Verification items for the finished model (mm, model axes). A direction names the side the tool comes from. Round coordinates to 2 decimals unless told otherwise and drop trailing zeros. Order: outer loops, then holes, each group sorted by start corner. A loop starts at its lowest first (then second) coordinate and runs counter-clockwise, first axis right, second up. Notation, with made-up numbers: M -1,-22.75 L 55,-22.75 A30 ccw 55,5.25 Z; hole C -1.5,-24 d10. An arc over 180 degrees is marked long. Use one line per item in the form item = value. Start each with the question number.
Item 1: Thickness scan on probe 1 along Z at (x, y) = (-33, 75); probe 2 along Y at (x, z) = (-4.85, 0.15); probe 3 along Y at (x, z) = (-4, 0). Record the ranges inside material, lowest first. Write a range as [from, to].
Item 2: Release check for a two-part mould opening along Z. For faces 5 (the flat face through (15, -19, 0)), 6 (the flat face through (33, 29, 14)), 7 (the flat face through (33, 51, 3.5)), 8 (the flat face through (0, 51, -2.5)) record: +Z half, -Z half, draft (parallel to the pull), parting line (faces both ways), or undercut.
Item 3: Cross-section at D-D on y = -17.5. Enter the section's corners in (x, z), then the cut area to 3 significant figures.
Item 4: Tool access check on faces 1 (the flat face through (-32, 66, 26)), 2 (the flat face through (-34, 73, 14)), 3 (the flat face through (11, 0, 0)), 4 (the flat face through (-15, -19, 0)). Record the directions out of +Z, -Z, +X, -X, +Y, -Y that give a thin tool (end or side, any length) a straight path to the whole face; none if there is none.
Item 5: Cross-section at C-C on z = 22. Enter the section's corners in (x, y).
Item 6: Go/stop test with flat-tipped pins: pin 1 Ø4 at (y, z) = (-15, -1) entering from -X; pin 2 Ø2.5 at (x, y) = (4.85, -24) entering from +Z; pin 3 Ø0.9 at (x, z) = (-33, 11) entering from -Y (3 decimals); pin 4 Ø2 at (x, y) = (-20, -5.5) entering from +Z. Record where each tip stops, or that it passes through.
Item 7: Cross-section at A-A on y = 49.5. Enter the section's corners in (x, z), then the cut area to 3 significant figures.
Item 8: Cross-section at B-B on x = -7.5. Enter the section's corners in (y, z), then the cut area to 3 significant figures.
from build123d import *

# Parameters (mm, degrees)
SKETCH1_R           = 1
SKETCH1_W           = 22
SKETCH1_H           = 44
BOSS_EXTRUDE1_DEPTH = 2.5
BOSS_EXTRUDE2_DEPTH = 34
CUT_EXTRUDE1_REACH  = 128.859
SKETCH3_R           = 1
SKETCH3_W           = 22
SKETCH3_H           = 44


with BuildPart() as part:
    # Sketch1 → Boss-Extrude1 (new, symmetric)
    with BuildSketch(Plane.XY):
        Polygon((-15, -29), (15, -29), (15, -9), (35, 21), (35, 101), (-35, 101), (-35, 21), (-15, -9), align=None)
        with Locations((-4.85, -24)):
            Circle(SKETCH1_R, mode=Mode.SUBTRACT)
        with Locations((4.85, -24)):
            Circle(SKETCH1_R, mode=Mode.SUBTRACT)
        with Locations((4.85, 24)):
            Circle(SKETCH1_R, mode=Mode.SUBTRACT)
        with Locations((-4.85, 24)):
            Circle(SKETCH1_R, mode=Mode.SUBTRACT)
        Rectangle(SKETCH1_W, SKETCH1_H, mode=Mode.SUBTRACT)
    extrude(amount=BOSS_EXTRUDE1_DEPTH, both=True)

    # Sketch2 → Boss-Extrude2 (add)
    with BuildSketch(Plane.XY.offset(-2.5)):
        Polygon((-35, 101), (-35, 21), (-32, 16.5), (-32, 98), (32, 98), (32, 16.5), (35, 21), (35, 101), align=None)
    extrude(amount=BOSS_EXTRUDE2_DEPTH)

    # Cut-Extrude1: up to this face of the body (flat: up to its plane)
    cut_extrude1_end = Plane(part.part.faces().sort_by_distance((35, 61, 14.5))[0])
    # Sketch3 → Cut-Extrude1 (cut, up to the picked face)
    with BuildSketch(Plane.ZY.offset(35), mode=Mode.PRIVATE) as cut_extrude1_sk1:
        with Locations(Location((9.65, 27, 0), (0, 0, 270))):
            Circle(SKETCH3_R)
    cut_extrude1_tool1 = split(extrude(cut_extrude1_sk1.sketch, amount=-CUT_EXTRUDE1_REACH, mode=Mode.PRIVATE), bisect_by=cut_extrude1_end, keep=Keep.BOTH, mode=Mode.PRIVATE)
    # Sketch3 → Cut-Extrude1 (cut, up to the picked face)
    with BuildSketch(Plane.ZY.offset(35), mode=Mode.PRIVATE) as cut_extrude1_sk2:
        with Locations(Location((19.35, 27, 0), (0, 0, 270))):
            Circle(SKETCH3_R)
    cut_extrude1_tool2 = split(extrude(cut_extrude1_sk2.sketch, amount=-CUT_EXTRUDE1_REACH, mode=Mode.PRIVATE), bisect_by=cut_extrude1_end, keep=Keep.BOTH, mode=Mode.PRIVATE)
    # Sketch3 → Cut-Extrude1 (cut, up to the picked face)
    with BuildSketch(Plane.ZY.offset(35), mode=Mode.PRIVATE) as cut_extrude1_sk3:
        with Locations(Location((19.35, 75, 0), (0, 0, 270))):
            Circle(SKETCH3_R)
    cut_extrude1_tool3 = split(extrude(cut_extrude1_sk3.sketch, amount=-CUT_EXTRUDE1_REACH, mode=Mode.PRIVATE), bisect_by=cut_extrude1_end, keep=Keep.BOTH, mode=Mode.PRIVATE)
    # Sketch3 → Cut-Extrude1 (cut, up to the picked face)
    with BuildSketch(Plane.ZY.offset(35), mode=Mode.PRIVATE) as cut_extrude1_sk4:
        with Locations(Location((9.65, 75, 0), (0, 0, 270))):
            Circle(SKETCH3_R)
    cut_extrude1_tool4 = split(extrude(cut_extrude1_sk4.sketch, amount=-CUT_EXTRUDE1_REACH, mode=Mode.PRIVATE), bisect_by=cut_extrude1_end, keep=Keep.BOTH, mode=Mode.PRIVATE)
    # Sketch3 → Cut-Extrude1 (cut, up to the picked face)
    with BuildSketch(Plane.ZY.offset(35), mode=Mode.PRIVATE) as cut_extrude1_sk5:
        with Locations((14.5, 51)):
            Rectangle(SKETCH3_W, SKETCH3_H)
    cut_extrude1_tool5 = split(extrude(cut_extrude1_sk5.sketch, amount=-CUT_EXTRUDE1_REACH, mode=Mode.PRIVATE), bisect_by=cut_extrude1_end, keep=Keep.BOTH, mode=Mode.PRIVATE)
    add(cut_extrude1_tool1.solids().sort_by(Axis((-35, 27, 9.65), (1, 0, 0)))[0], mode=Mode.SUBTRACT)
    add(cut_extrude1_tool2.solids().sort_by(Axis((-35, 27, 19.35), (1, 0, 0)))[0], mode=Mode.SUBTRACT)
    add(cut_extrude1_tool3.solids().sort_by(Axis((-35, 75, 19.35), (1, 0, 0)))[0], mode=Mode.SUBTRACT)
    add(cut_extrude1_tool4.solids().sort_by(Axis((-35, 75, 9.65), (1, 0, 0)))[0], mode=Mode.SUBTRACT)
    add(cut_extrude1_tool5.solids().sort_by(Axis((-35, 51, 14.5), (1, 0, 0)))[0], mode=Mode.SUBTRACT)


solid = part.part
Output values:
q1.probe_1 = [-2.5, 8.65], [10.65, 18.35], [20.35, 31.5]
q1.probe_2 = [-29, -25], [-23, -22], [22, 23], [25, 101]
q1.probe_3 = [-29, -24.53], [-23.47, -22], [22, 23.47], [24.53, 101]
q2.face_5 = draft
q2.face_6 = undercut
q2.face_7 = undercut
q2.face_8 = -Z half
q3.outline = M -15,-2.5 L -11,-2.5 L -11,2.5 L -15,2.5 Z; M 11,-2.5 L 15,-2.5 L 15,2.5 L 11,2.5 Z
q3.area = 40.0 mm2
q4.face_1 = +Z, -Y
q4.face_2 = +X, -X
q4.face_3 = +Z, -Z
q4.face_4 = +Z, -Z, -X, -Y
q5.outline = M -35,21 L -32,16.5 L -32,29 L -35,29 Z; M -35,73 L -32,73 L -32,98 L 32,98 L 32,73 L 35,73 L 35,101 L -35,101 Z; M 32,16.5 L 35,21 L 35,29 L 32,29 Z
q6.pin_1 = -15
q6.pin_2 = 2.5
q6.pin_3 = 17.325
q6.pin_4 = through
q7.outline = M -35,-2.5 L 35,-2.5 L 35,3.5 L 32,3.5 L 32,2.5 L -32,2.5 L -32,3.5 L -35,3.5 Z; M -35,25.5 L -32,25.5 L -32,31.5 L -35,31.5 Z; M 32,25.5 L 35,25.5 L 35,31.5 L 32,31.5 Z
q7.area = 392 mm2
q8.outline = M -29,-2.5 L -22,-2.5 L -22,2.5 L -29,2.5 Z; M 22,-2.5 L 101,-2.5 L 101,31.5 L 98,31.5 L 98,2.5 L 22,2.5 Z
q8.area = 517 mm2
